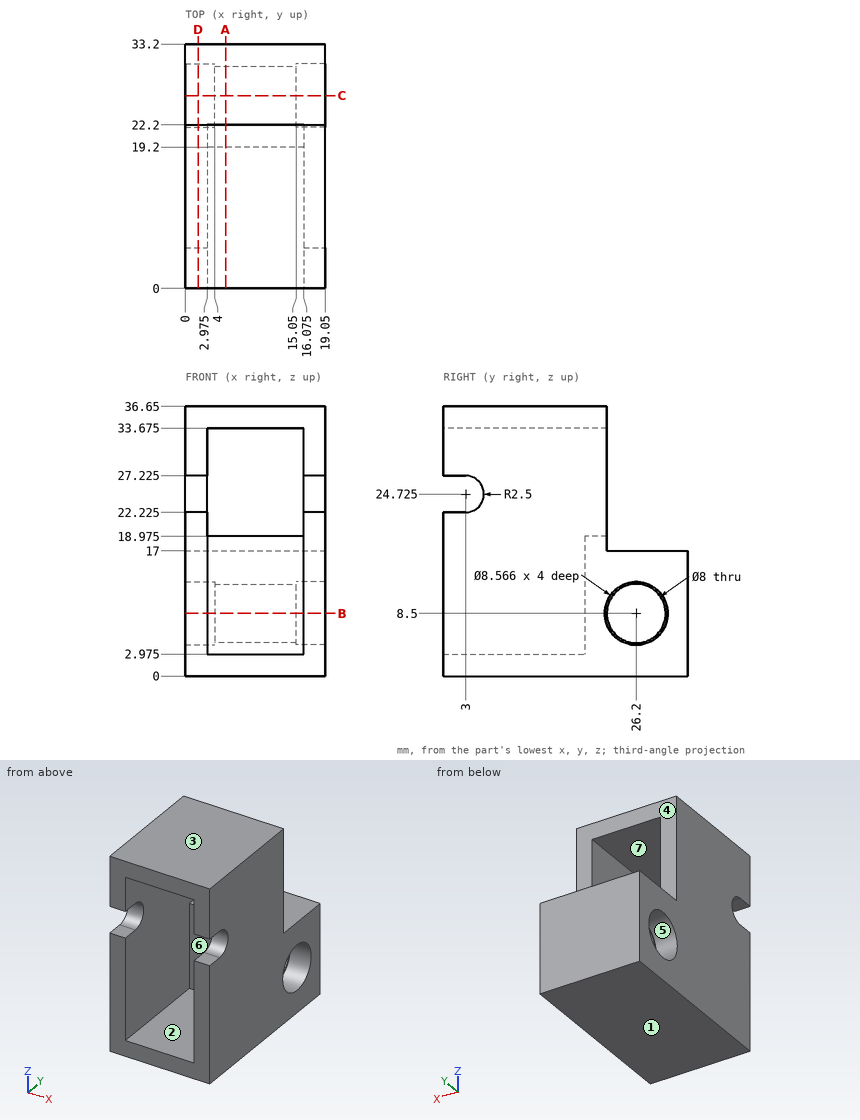
Answer from the drawing. Dimensions are ordinates in mm from the lowest x, y and z of the part. A direction names the side the tool comes from. Give positions to 0.01 mm unless a question says otherwise; leave off trailing zeros. Write each loop counter-clockwise with the first axis right and the second up, starting at its lowest first coordinate (ties: lowest second). Pieces come first, ordered by that corner, then holes.
1) Find the intervals of material crossed by L1, parallel to Z at x = 17.3, y = 26.2; L2, parallel to Z at x = 14, y = 2 (3 decimals); L3, parallel to X at y = 12, z = 13.5 (3 decimals), in increasing order.
2) A tool of negligible diameter and unlimited length cuts with its end or side. For the marked faces 4, 5, 6 and 7, from which of +Z, -Z, +X, -X, +Y, -Y can it reach the whole face along a straight path? Write none if from no direction.
3) Given P1, Ø3.5, axis at x = 10, y = 29, coming from the +Z side; P2, Ø10, axis at x = 11, z = 23.5, coming from the +Y side, each flat-ended and moving along its own axis, determine where each tip first touches the part or whether it passes through.
4) For a pull along Z with two mould halves and no side action, classify the marked faces 1, 2 and 3 as pulls with the +Z half, pulls with the -Z half, needs draft (parallel to the pull), parting line crosses it, or undercut.
5) Section B-B (z = 8.5) is taken. Write down the section's boundary in (x, y) (3 decimals), and give its area (3 significant figures).
6) Section C-C (y = 26.2) is taken. Write down the section's boundary in (x, z), and give its area (3 significant figures).
7) Section A-A (x = 5.5) is taken. Write down the section's boundary in (y, z) (3 decimals), and give its area (3 significant figures).
8) Section D-D (x = 1.75) is taken. Write down the section's boundary in (y, z) (3 decimals), and give its area (3 significant figures).
Response:
1. L1: z = 0 to 4.22, 12.78 to 17
1. L2: z = 0 to 2.975, 33.675 to 36.65
1. L3: x = 0 to 2.975, 16.075 to 19.05
2. face 4: +Z, +X, -X, +Y
2. face 5: -X
2. face 6: -Y
2. face 7: +Y, -Y
3. P1: stops at z = 17
3. P2: stops at y = 22.2
4. face 1: pulls with the -Z half
4. face 2: undercut
4. face 3: pulls with the +Z half
5. outline: (0, 0) - (2.975, 0) - (2.975, 19.2) - (16.075, 19.2) - (16.075, 0) - (19.05, 0) - (19.05, 21.917) - (15.05, 21.917) - (15.05, 22.2) - (4, 22.2) - (4, 21.917) - (0, 21.917) - close; (0, 30.483) - (4, 30.483) - (4, 30.2) - (15.05, 30.2) - (15.05, 30.483) - (19.05, 30.483) - (19.05, 33.2) - (0, 33.2) - close
5. area: 224 mm2
6. outline: (0, 0) - (19.05, 0) - (19.05, 4.22) - (15.05, 4.22) - (15.05, 4.5) - (4, 4.5) - (4, 4.22) - (0, 4.22) - close; (0, 12.78) - (4, 12.78) - (4, 12.5) - (15.05, 12.5) - (15.05, 12.78) - (19.05, 12.78) - (19.05, 17) - (0, 17) - close
6. area: 167 mm2
7. outline: (0, 0) - (33.2, 0) - (33.2, 17) - (22.2, 17) - (22.2, 18.975) - (19.2, 18.975) - (19.2, 2.975) - (0, 2.975) - close; (0, 33.675) - (22.2, 33.675) - (22.2, 36.65) - (0, 36.65) - close; hole circle Ø8 at (26.2, 8.5)
7. area: 317 mm2
8. outline: (0, 0) - (33.2, 0) - (33.2, 17) - (22.2, 17) - (22.2, 36.65) - (0, 36.65) - (0, 27.225) - (3, 27.225) arc R2.5 cw to (3, 22.225) - (0, 22.225) - close; hole circle Ø8.566 at (26.2, 8.5)
8. area: 918 mm2
